Read the model definition and answer for the solid it produces. Units are mm, in the model's axes. A direction names the side the tool comes from. Give positions to 0.01 mm unless a question says otherwise; leave off trailing zeros. Order: outer loops, then holes, each group sorted by start corner. A loop starts at its lowest first (then second) coordinate and runs counter-clockwise, first axis right, second up. Notation, with made-up numbers: (28, 9) - (57, 9) arc R31 ccw to (57, 44) - close; hole circle Ø9 at (-17.5, 48.25). An arc over 180 degrees is marked (long way). Write each question's results on one line, items separated by ' | '.
from build123d import *

# Parameters (mm, degrees)
F1_DEPTH = 1.5
F2_R     = 2.5
F3_DEPTH = 72.5
F4_DEPTH = 67


with BuildPart() as f1:
    # F0 (on Top) → F1 (new body, symmetric)
    with BuildSketch(Plane.XY):
        with BuildLine():
            Line((50, 25), (-50, 25))
            ThreePointArc((-50, 25), (-64.1421356237, 19.1421356237), (-70, 5))
            Line((-70, 5), (-70, -5))
            ThreePointArc((-70, -5), (-64.1421356237, -19.1421356237), (-50, -25))
            Line((-50, -25), (50, -25))
            ThreePointArc((50, -25), (64.1421356237, -19.1421356237), (70, -5))
            Line((70, -5), (70, 5))
            ThreePointArc((70, 5), (64.1421356237, 19.1421356237), (50, 25))
        make_face()
        with BuildLine():
            Line((-67, -5), (-67, 5))
            ThreePointArc((-67, 5), (-62.0208152802, 17.0208152802), (-50, 22))
            Line((-50, 22), (50, 22))
            ThreePointArc((50, 22), (62.0208152802, 17.0208152802), (67, 5))
            Line((67, 5), (67, -5))
            ThreePointArc((67, -5), (62.0208152802, -17.0208152802), (50, -22))
            Line((50, -22), (-50, -22))
            ThreePointArc((-50, -22), (-62.0208152802, -17.0208152802), (-67, -5))
        make_face(mode=Mode.SUBTRACT)
    extrude(amount=F1_DEPTH, both=True)

    # F2 (on Right) → F3 (join)
    with BuildSketch(Plane.YZ):
        Circle(F2_R)
    extrude(amount=F3_DEPTH)

    # F2 (on Right) → F4 (cut, through all)
    with BuildSketch(Plane.YZ):
        Circle(F2_R)
    extrude(amount=F4_DEPTH, mode=Mode.SUBTRACT)

    # F5: F1 across plane


with BuildPart() as f1_1:
    add(f1.part)
    add(f1.part.mirror(Plane.YZ))


solid = f1_1.part
(1) Each of these flat-tipped pins is pushed along its axis until it touches: pin 1 (0.9 mm diameter, centred on y = 3.5, z = -0.5, fed in from +X); pin 2 (1.5 mm diameter, centred on y = -3.5, z = -0.5, fed in from -X); pin 3 (18.5 mm diameter, centred on x = 28.5, y = 14, fed in from +Z); pin 4 (11.5 mm diameter, centred on x = -9.5, y = -12, fed in from +Z). Where does it stop, or does it pass through?
Conclusion:
pin 1: x = 70 | pin 2: x = -70 | pin 3: z = 1.5 | pin 4: through
(2) Section C-C (x = -41.5) is taken. Give the vertices of the cut face in (y, z), plus the area to 3 significant figures.
Conclusion:
outline: (-25, -1.5) - (-22, -1.5) - (-22, 1.5) - (-25, 1.5) - close; (22, -1.5) - (25, -1.5) - (25, 1.5) - (22, 1.5) - close | area: 18.0 mm^2
(3) Section A-A (y = 0) is taken. Give the vertices of the cut face in (x, z), plus the area to 3 significant figures.
Conclusion:
outline: (-72.5, -2.5) - (-67, -2.5) - (-67, 2.5) - (-72.5, 2.5) - close; (67, -2.5) - (72.5, -2.5) - (72.5, 2.5) - (67, 2.5) - close | area: 55.0 mm^2
(4) The mould has two halves that part along X. Classify faces 1 (the face through (70, -4, 0)), 2 (the face through (-1, 22, 0)), 3 (the face through (0, -23, 1.5)): pulls with the +X half, pulls with the -X half, needs draft (parallel to the pull), parting line crosses it, or undercut.
Conclusion:
face 1: pulls with the +X half | face 2: undercut | face 3: needs draft
(5) For faces 4 (the face through (70.3, -2.5, 0.1)), 5 (the face through (-70.3, -2.5, 0.1)), 6 (the face through (0, 23, 1.5)), 7 (the face through (-62.15, 16.89, 0.02)), determine the directions among +Z, -Z, +X, -X, +Y, -Y from which every point of the face is accessible in a straight line to the end or side of a thin tool.
Conclusion:
face 4: +X | face 5: -X | face 6: +Z, +X, -X, +Y | face 7: +Z, -Z
(6) Consider probe 1 along Y at (x, z) = (34, -0.75); probe 2 along X at (y, z) = (-1.5, 0.8); probe 3 along X at (y, z) = (-5, 0.35). Determine where each line is inside the solid, lowest interval first. Write a range as [from, to].
Conclusion:
probe 1: [-25, -22], [22, 25] | probe 2: [-72.5, -67], [67, 72.5] | probe 3: [-70, -67], [67, 70]
(7) Section B-B (z = 0) is taken. Give the vertices of the cut face in (x, y), plus the area to 3 significant figures.
Conclusion:
outline: (-72.5, -2.5) - (-70, -2.5) - (-70, -5) arc R20 ccw to (-50, -25) - (50, -25) arc R20 ccw to (70, -5) - (70, -2.5) - (72.5, -2.5) - (72.5, 2.5) - (70, 2.5) - (70, 5) arc R20 ccw to (50, 25) - (-50, 25) arc R20 ccw to (-70, 5) - (-70, 2.5) - (-72.5, 2.5) - close; hole (-67, -5) arc R17 ccw to (-50, -22) - (50, -22) arc R17 ccw to (67, -5) - (67, 5) arc R17 ccw to (50, 22) - (-50, 22) arc R17 ccw to (-67, 5) - close | area: 1,030 mm^2
